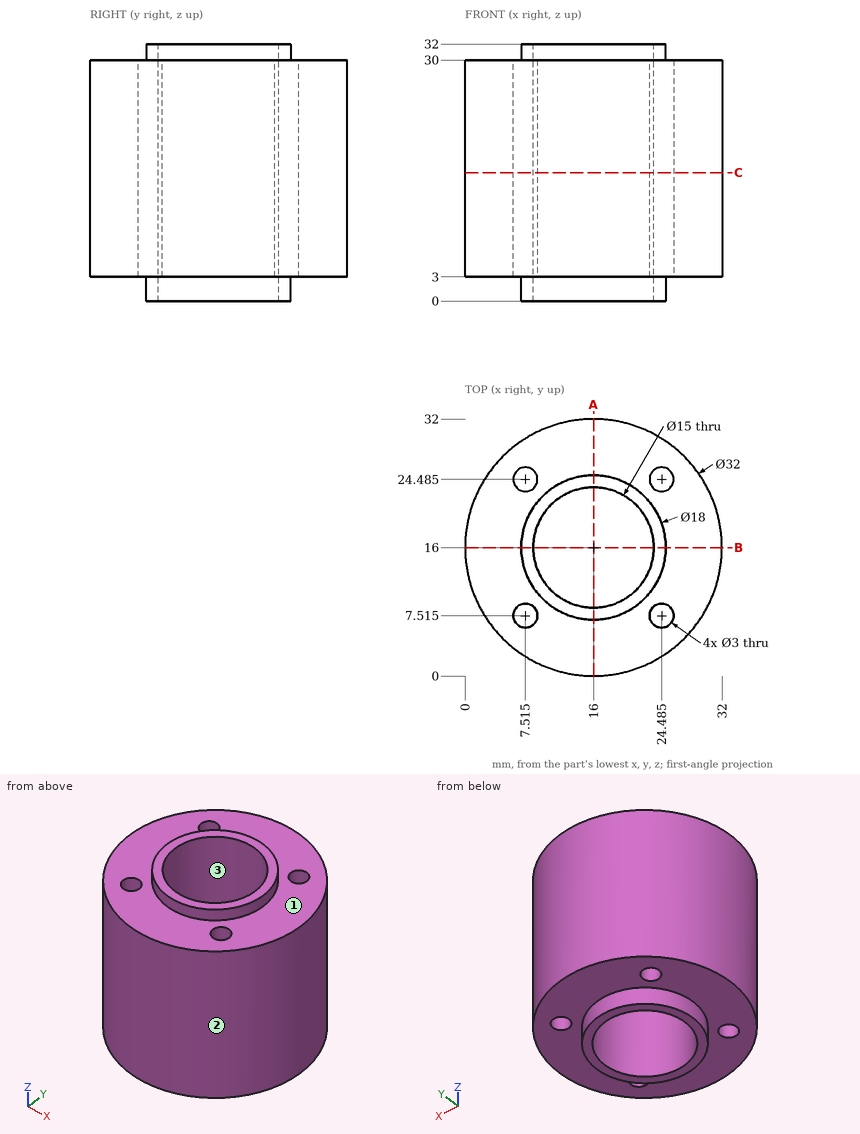
Can you work these out from the drawing? Everything is in mm from the part's minimum corner. Round coordinates to 2 decimals unless told otherwise and drop trailing zeros. Loops run counter-clockwise (first coordinate to the right, second up) from the corner with the lowest first, then second, coordinate; pieces in that order, holes last. Notation, with made-up numbers: (84, 13) -> (124, 13) arc R16 cw to (124, 22) -> close; hole circle Ø8 at (-17.75, 46.25). An arc over 180 degrees is marked (long way). Put each result on its own line as item: value.
Q1. Thinking about a two-plate mould opening in X: for the marked faces 1, 2 and 3, which applies, pulls with the +X half, pulls with the -X half, needs draft (parallel to the pull), parting line crosses it, or undercut?
Checks:
face 1: needs draft
face 2: parting line crosses it
face 3: undercut
Q2. I want a section at C-C on z = 16. Write out the boundary of the cut face in (x, y) (1 decimal).
Checks:
outline: circle Ø32 at (16, 16); hole circle Ø3 at (7.5, 7.5); hole circle Ø3 at (7.5, 24.5); hole circle Ø15 at (16, 16); hole circle Ø3 at (24.5, 7.5); hole circle Ø3 at (24.5, 24.5)
Q3. For pin 1 Ø6 at (x, z) = (5.5, 28) entering from -Y; pin 2 Ø6 at (y, z) = (28, 27.5) entering from -X; pin 3 Ø2.5 at (x, y) = (24.49, 7.51) entering from -Z; pin 4 Ø4 at (y, z) = (27, 6.5) entering from +X, each with a flat end and sliding along its axis, tell me the tip position at first contact or that it passes through.
Checks:
pin 1: y = 1.87
pin 2: x = 2.77
pin 3: through
pin 4: x = 29.23
Q4. Please list where these lines run through material, in increasing order: line 1 (Y direction, x = 8, z = 12) (1 decimal); line 2 (Z direction, x = 18, y = 5); line 3 (Y direction, x = 14.5, z = 4). Write a range as from..to.
Checks:
line 1: 2.1..6.1, 8.9..23.1, 25.9..29.9
line 2: 3..30
line 3: 0.07..8.65, 23.35..31.93
Q5. I want a section at A-A on x = 16. Write out the boundary of the cut face in (y, z), and give its area (3 significant figures).
Checks:
outline: (0, 3) -> (7, 3) -> (7, 0) -> (8.5, 0) -> (8.5, 32) -> (7, 32) -> (7, 30) -> (0, 30) -> close; (23.5, 0) -> (25, 0) -> (25, 3) -> (32, 3) -> (32, 30) -> (25, 30) -> (25, 32) -> (23.5, 32) -> close
area: 474 mm2
